The listing builds one solid part. Answer for the finished solid, in the listing's coordinates (mm). A direction names the side the tool comes from. Round coordinates to 2 decimals unless told otherwise and drop trailing zeros. Loops run counter-clockwise (first coordinate to the right, second up) from the corner with the lowest first, then second, coordinate; pieces in that order, holes last. Notation, with made-up numbers: (56, -15.75) -> (101, -15.75) arc R6 ccw to (101, -4.75) -> close; hole circle Ø1 at (79, -37). An arc over 180 degrees is marked (long way). Use a Markdown table: item, result. Add a question column.
Q1. Consider line 1 (Y direction, x = -15, z = 2.55); line 2 (Z direction, x = 4, y = 4); line 3 (Z direction, x = -17.5, y = -6). Determine where each line is inside the solid, lowest interval first.
Q2. Section A-A on x = -15 is taken. Give the vertices of the cut face in (y, z), then the cut area to 3 significant figures.
Q3. For a pull along X with two mould halves and no side action, classify faces 1 (the flat face through (20, 0, 2)), 2 (the cylindrical face through (-0.683, -0.14, 15.455)), 3 (the flat face through (0, -10, 3)) as released by +X, released by -X, zero draft, split by the parting line, or undercut.
Q4. Section B-B on y = 0 is taken. Give the number of separate pieces and of enclosed holes in the cut face, then the cut area to 3 significant figures.
Q5. Which of the six approach directions +Z, -Z, +X, -X, +Y, -Y give full straight-line access (tool end or side, diameter ignored) to faces 4 (the flat face through (-10, 0, 7)), 5 (the flat face through (13.8, 2.4, 5)), 6 (the cylindrical face through (12.5, 0.1, 2.5))?
Q6. Section C-C on z = 7 is taken. Give the vertices of the cut face in (x, y), then the cut area to 3 significant figures.
Q7. Given pin 1 Ø1.5 at (y, z) = (-2, 7) entering from -X; pin 2 Ø10 at (x, y) = (13, -7) entering from +Z; pin 3 Ø11 at (x, y) = (17, -4.5) entering from +Z; pin 4 Ø3 at (x, y) = (-15, 0) entering from +Z, each flat-ended and moving along its own axis, determine where each tip first touches the part or whether it passes through.
from build123d import *

# Parameters (mm, degrees)
F0_W     = 40
F0_H     = 20
F0_R     = 2.5
F1_DEPTH = 5
F2_W     = 20
F2_H     = 20
F3_DEPTH = 15
F4_R     = 5.25
F5_DEPTH = 25
F6_R     = 9.99999


# Not quite as in the source:
# - a fillet or chamfer is up to 0.001 mm smaller than in the source, because OpenCascade refuses the exact size


with BuildPart() as f1:
    # F0 (on Top) → F1 (new body)
    with BuildSketch(Plane.XY):
        Rectangle(F0_W, F0_H)
        with Locations((-15, 0)):
            Circle(F0_R, mode=Mode.SUBTRACT)
        with Locations((15, 0)):
            Circle(F0_R, mode=Mode.SUBTRACT)
    extrude(amount=F1_DEPTH)

    # F2 (on face) → F3 (join)
    with BuildSketch(Plane.XY.offset(5)):
        Rectangle(F2_W, F2_H)
    extrude(amount=F3_DEPTH)

    # F4 (on face) → F5 (cut)
    with BuildSketch(Plane.XZ.offset(10)):
        with Locations((0, 10.25)):
            Circle(F4_R)
    extrude(amount=-F5_DEPTH, mode=Mode.SUBTRACT)

    # F6 (radius 10 in the source; OpenCascade refuses exactly that, so slightly less here)
    f6_edges = [f1.edges().sort_by_distance(p)[0] for p in [
        (-10, 0, 20),
        (10, 0, 20),
    ]]
    fillet(f6_edges, radius=F6_R)


solid = f1.part
Checked values:
| question | item | result |
|---|---|---|
| 1 | line 1 | y = -10 to -2.5, 2.5 to 10 |
| 1 | line 2 | z = 0 to 6.85, 13.65 to 19.17 |
| 1 | line 3 | z = 0 to 5 |
| 2 | outline | (-10, 0) -> (-2.5, 0) -> (-2.5, 5) -> (-10, 5) -> close; (2.5, 0) -> (10, 0) -> (10, 5) -> (2.5, 5) -> close |
| 2 | area | 75.0 mm2 |
| 3 | face 1 | released by +X |
| 3 | face 2 | undercut |
| 3 | face 3 | zero draft |
| 4 | separate pieces | 3 |
| 4 | enclosed holes | 1 |
| 4 | area | 320 mm2 |
| 5 | face 4 | +Z, -X, +Y, -Y |
| 5 | face 5 | +Z, +X, +Y, -Y |
| 5 | face 6 | +Z, -Z |
| 6 | outline | (-10, -10) -> (-4.12, -10) -> (-4.12, 10) -> (-10, 10) -> close; (4.12, -10) -> (10, -10) -> (10, 10) -> (4.12, 10) -> close |
| 6 | area | 235 mm2 |
| 7 | pin 1 | stops at x = -10 |
| 7 | pin 2 | stops at z = 16 |
| 7 | pin 3 | stops at z = 5 |
| 7 | pin 4 | passes through |
